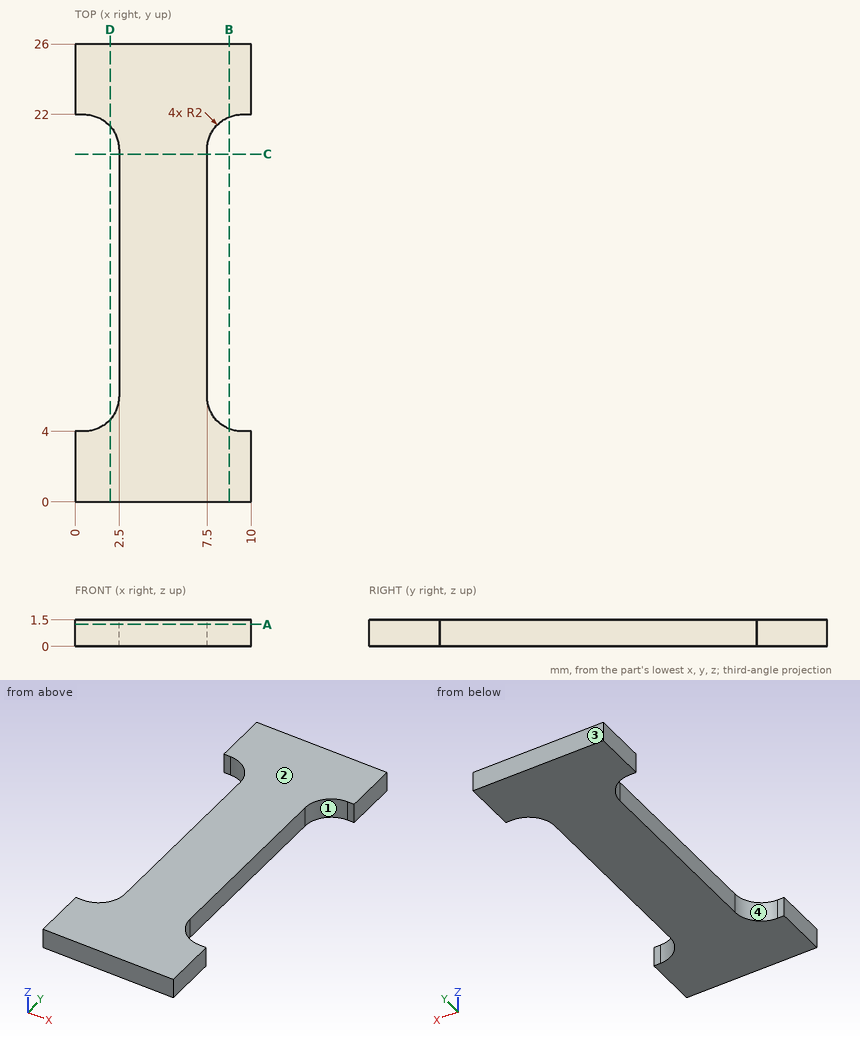
Geometry check sheet. Reference: drawing and pictorial views, mm from the part's lowest x, y, z. Round coordinates to 2 decimals unless told otherwise and drop trailing zeros. Write each loop counter-clockwise with the first axis right and the second up, starting at its lowest first coordinate (ties: lowest second). Pieces come first, ordered by that corner, then holes. Notation, with made-up numbers: (32.5, 84.5) -> (69.5, 84.5) arc R20 ccw to (69.5, 107.5) -> close; hole circle Ø9 at (37.5, 40). An arc over 180 degrees is marked (long way). Answer as CSV lines item,"result". Start each with the question number.
1) Section check A-A on z = 1.25. Enter the section's corners in (x, y).
2) Material ranges on line 1 (Y direction, x = 9.5, z = 1.45); line 2 (X direction, y = 13, z = 0.5); line 3 (Y direction, x = 1.75, z = 0.3), recorded low to high. Write a range as from..to.
3) Section check C-C on y = 19.75. Enter the section's corners in (x, z).
4) Section check D-D on x = 2. Enter the section's corners in (y, z).
5) Release check for a two-part mould opening along Y. For the marked faces 1, 2, 3 and 4 record: pulls with the +Y half, pulls with the -Y half, needs draft (parallel to the pull), parting line crosses it, or undercut.
6) Section check B-B on x = 8.75. Enter the section's corners in (y, z).
Found:
1,outline,"(0, 0) -> (10, 0) -> (10, 4) -> (9.5, 4) arc R2 cw to (7.5, 6) -> (7.5, 20) arc R2 cw to (9.5, 22) -> (10, 22) -> (10, 26) -> (0, 26) -> (0, 22) -> (0.5, 22) arc R2 cw to (2.5, 20) -> (2.5, 6) arc R2 cw to (0.5, 4) -> (0, 4) -> close"
2,line 1,"y = 0..4, 22..26"
2,line 2,"x = 2.5..7.5"
2,line 3,"y = 0..4.44, 21.56..26"
3,outline,"(2.5, 0) -> (7.5, 0) -> (7.5, 1.5) -> (2.5, 1.5) -> close"
4,outline,"(0, 0) -> (4.68, 0) -> (4.68, 1.5) -> (0, 1.5) -> close; (21.32, 0) -> (26, 0) -> (26, 1.5) -> (21.32, 1.5) -> close"
5,face 1,"undercut"
5,face 2,"needs draft"
5,face 3,"pulls with the +Y half"
5,face 4,"undercut"
6,outline,"(0, 0) -> (4.15, 0) -> (4.15, 1.5) -> (0, 1.5) -> close; (21.85, 0) -> (26, 0) -> (26, 1.5) -> (21.85, 1.5) -> close"
